Part print with two shaded views. Sizes in mm from the minimum x, y, z corner. A direction names the side the tool comes from. Round coordinates to 2 decimals unless told otherwise and drop trailing zeros. Write each loop counter-clockwise with the first axis right and the second up, starting at its lowest first coordinate (ties: lowest second). Pieces come first, ordered by that corner, then holes. Notation, with made-up numbers: (88.5, 62.25) -> (128.5, 62.25) arc R27 cw to (128.5, 93.25) -> close; hole circle Ø10 at (19, -39). An arc over 180 degrees is marked (long way). Answer as CSV lines item,"result".
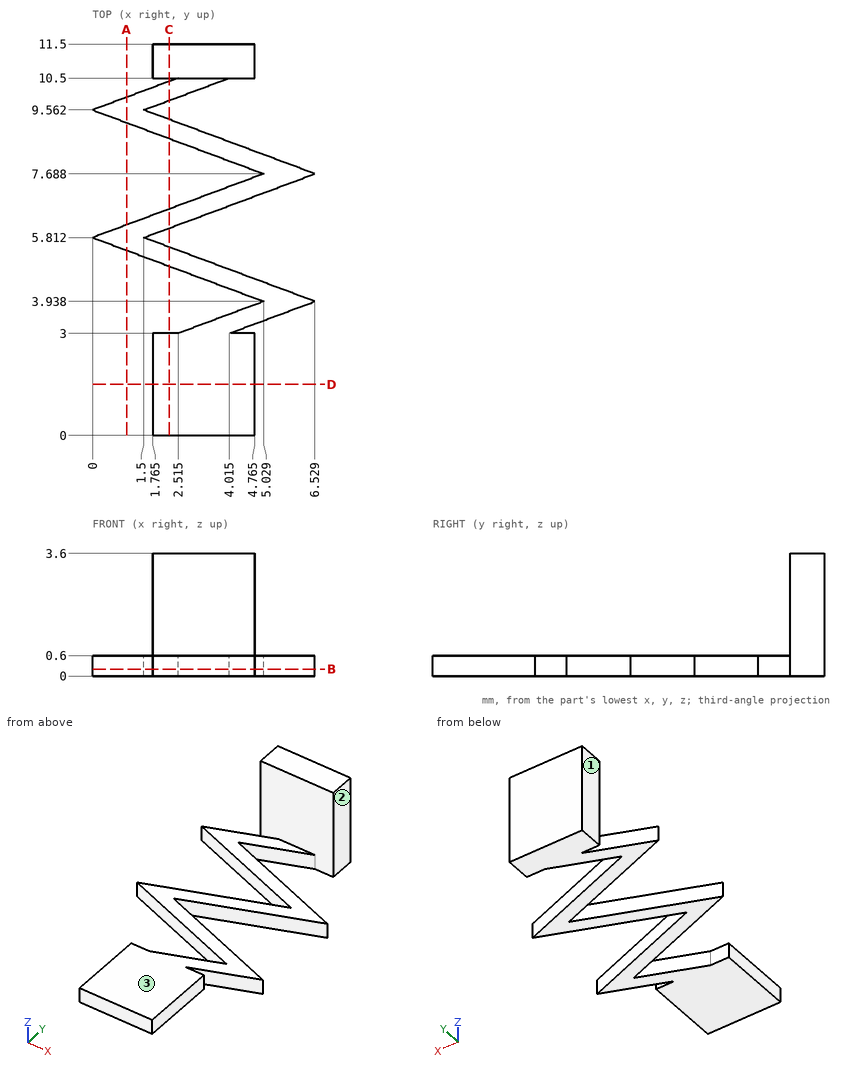
1. Cut at B-B, the plane z = 0.2. Write the cut outline in (x, y) (1 decimal).
Results found:
outline,"(0, 5.8) -> (5, 3.9) -> (2.5, 3) -> (1.8, 3) -> (1.8, 0) -> (4.8, 0) -> (4.8, 3) -> (4, 3) -> (6.5, 3.9) -> (1.5, 5.8) -> (6.5, 7.7) -> (1.5, 9.6) -> (4, 10.5) -> (4.8, 10.5) -> (4.8, 11.5) -> (1.8, 11.5) -> (1.8, 10.5) -> (2.5, 10.5) -> (0, 9.6) -> (5, 7.7) -> close"
2. Cut at C-C, the plane x = 2.25. Write the cut outline in (y, z).
Results found:
outline,"(0, 0) -> (3, 0) -> (3, 0.6) -> (0, 0.6) -> close; (4.97, 0) -> (5.53, 0) -> (5.53, 0.6) -> (4.97, 0.6) -> close; (6.09, 0) -> (6.65, 0) -> (6.65, 0.6) -> (6.09, 0.6) -> close; (8.72, 0) -> (9.28, 0) -> (9.28, 0.6) -> (8.72, 0.6) -> close; (9.84, 0) -> (10.4, 0) -> (10.4, 0.6) -> (9.84, 0.6) -> close; (10.5, 0) -> (11.5, 0) -> (11.5, 3.6) -> (10.5, 3.6) -> close"
3. Drop flat-ended pins along their axis: pin 1 Ø1.5 at (x, z) = (2.5, 2) entering from -Y; pin 2 Ø0.5 at (y, z) = (11, 2.5) entering from -X (1 decimal); pin 3 Ø1 at (y, z) = (8.5, 2) entering from +X. Give the stop position or say it passes through.
Results found:
pin 1,"stops at y = 10.5"
pin 2,"stops at x = 1.8"
pin 3,"passes through"
4. Cut at A-A, the plane x = 1. Write the cut outline in (y, z) (1 decimal).
Results found:
outline,"(5.4, 0) -> (6.2, 0) -> (6.2, 0.6) -> (5.4, 0.6) -> close; (9.2, 0) -> (9.9, 0) -> (9.9, 0.6) -> (9.2, 0.6) -> close"
5. Which spindle directions (+Z, -Z, +X, -X, +Y, -Y) get a long thin tool onto all of the face, cutting with end or side? Do the marked faces 1, 2 and 3. Say none if no direction does.
Results found:
face 1,"+Z, -Z, -X, +Y"
face 2,"+Z, -Z, +X, +Y"
face 3,"+Z, +X, -X, -Y"
6. Cut at D-D, the plane y = 1.5. Write the cut outline in (x, z) (1 decimal).
Results found:
outline,"(1.8, 0) -> (4.8, 0) -> (4.8, 0.6) -> (1.8, 0.6) -> close"
7. Probe line 1 along Y through (x, z) = (3.5, 0.35); line 2 along Z through (x, y) = (2.5, 2); line 3 along Y through (x, z) = (2.5, 1.2). List the from-to ranges inside material, lowest first.
Results found:
line 1,"y = 0 to 3.37, 4.51 to 5.07, 6.56 to 7.12, 8.26 to 8.82, 10.31 to 11.5"
line 2,"z = 0 to 0.6"
line 3,"y = 10.5 to 11.5"
